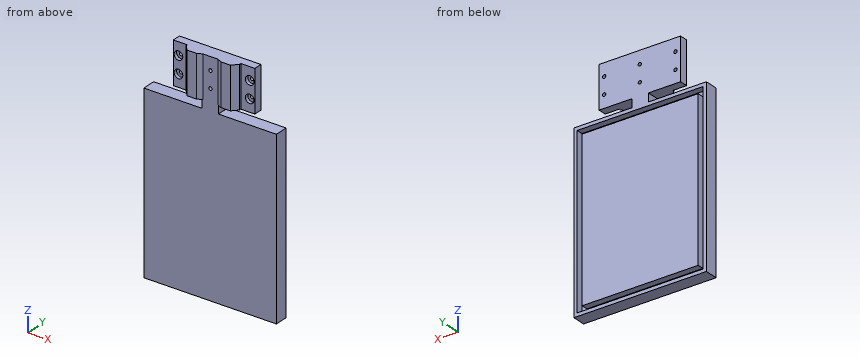
from build123d import *

# Parameters (mm, degrees)
BOSS_EXTRUDE2_DEPTH = 25.3
SKETCH3_R           = 1
CUT_EXTRUDE1_DEPTH  = 37.183559803
SKETCH4_R           = 1
CUT_EXTRUDE2_DEPTH  = 36.640566774
SKETCH5_R           = 2.6
CUT_EXTRUDE3_DEPTH  = 2
SKETCH7_W           = 10
SKETCH7_H           = 8
BOSS_EXTRUDE4_DEPTH = 5
SKETCH8_W           = 80
SKETCH8_H           = 8
BOSS_EXTRUDE5_DEPTH = 105
SKETCH9_W           = 76
SKETCH9_H           = 101
SKETCH9_W_2         = 70
SKETCH9_H_2         = 95
CUT_EXTRUDE4_DEPTH  = 4


with BuildPart() as part:
    # Sketch2 → Boss-Extrude2 (new body)
    with BuildSketch(Plane.XY):
        Polygon((4.5, 3.4), (-4.5, 3.4), (-7.5, 2), (-13.1, 2), (-16.1, 5.4), (-16.1, 6.4), (-24.6, 6.4), (-24.6, 11.4), (24.6, 11.4), (24.6, 6.4), (16.1, 6.4), (16.1, 5.4), (13.1, 2), (7.5, 2), align=None)
    extrude(amount=BOSS_EXTRUDE2_DEPTH)

    # Sketch3 → Cut-Extrude1 (cut, through all)
    with BuildSketch(Plane.XZ.offset(-3.4)):
        with Locations(Location((0, 17.55, 0), (0, 0, 270))):
            Circle(SKETCH3_R)
        with Locations(Location((0, 7.55, 0), (0, 0, 90))):
            Circle(SKETCH3_R)
    extrude(amount=-CUT_EXTRUDE1_DEPTH, mode=Mode.SUBTRACT)

    # Sketch4 → Cut-Extrude2 (cut, through all)
    with BuildSketch(Plane.XZ.offset(-6.4)):
        with Locations(Location((-21.5, 17.65, 0), (0, 0, 270))):
            Circle(SKETCH4_R)
        with Locations(Location((21.5, 17.65, 0), (0, 0, 90))):
            Circle(SKETCH4_R)
        with Locations(Location((-21.5, 7.65, 0), (0, 0, 270))):
            Circle(SKETCH4_R)
        with Locations(Location((21.5, 7.65, 0), (0, 0, 90))):
            Circle(SKETCH4_R)
    extrude(amount=-CUT_EXTRUDE2_DEPTH, mode=Mode.SUBTRACT)

    # Sketch5 → Cut-Extrude3 (cut)
    with BuildSketch(Plane.XZ.offset(-6.4)):
        with Locations(Location((-21.5, 17.65, 0), (0, 0, 270))):
            Circle(SKETCH5_R)
        with Locations(Location((-21.5, 7.45, 0), (0, 0, 90))):
            Circle(SKETCH5_R)
        with Locations(Location((21.5, 7.45, 0), (0, 0, 270))):
            Circle(SKETCH5_R)
        with Locations(Location((21.5, 17.65, 0), (0, 0, 90))):
            Circle(SKETCH5_R)
    extrude(amount=-CUT_EXTRUDE3_DEPTH, mode=Mode.SUBTRACT)

    # Sketch7 → Boss-Extrude4 (add)
    with BuildSketch(Plane(origin=(0, 0, 0), x_dir=(-1, 0, 0), z_dir=(0, 0, -1))):
        with Locations((0.191701822, 7.4)):
            Rectangle(SKETCH7_W, SKETCH7_H)
    extrude(amount=BOSS_EXTRUDE4_DEPTH)

    # Sketch8 → Boss-Extrude5 (add)
    with BuildSketch(Plane(origin=(0, 0, -5), x_dir=(-1, 0, 0), z_dir=(0, 0, -1))):
        with Locations((0.191701822, 7.4)):
            Rectangle(SKETCH8_W, SKETCH8_H)
    extrude(amount=BOSS_EXTRUDE5_DEPTH)

    # Sketch9 → Cut-Extrude4 (cut)
    with BuildSketch(Plane(origin=(0, 11.4, 0), x_dir=(1, 0, 0), z_dir=(0, 1, 0))):
        with Locations((-0.191701822, 57.5)):
            Rectangle(SKETCH9_W, SKETCH9_H)
        with Locations((-0.191701822, 57.5)):
            Rectangle(SKETCH9_W_2, SKETCH9_H_2, mode=Mode.SUBTRACT)
    extrude(amount=-CUT_EXTRUDE4_DEPTH, mode=Mode.SUBTRACT)


solid = part.part
Design review of the part built by this model. Coordinates are the model's own, in mm. Coordinates: 2 decimals unless noted, no trailing zeros. Order: outer loops, then holes, each group sorted by start corner. A loop starts at its lowest first (then second) coordinate and runs counter-clockwise, first axis right, second up. Notation, with made-up numbers: (13.25, 9.25) -> (48.25, 9.25) arc R13 cw to (48.25, 16.25) -> close; hole circle Ø5 at (18.25, 31). An arc over 180 degrees is marked (long way). One line per item, written item: value.
1) We need section C-C, the plane x = 32. Give the boundary of the cut face in (y, z).
Output values:
outline: (3.4, -110) -> (11.4, -110) -> (11.4, -108) -> (7.4, -108) -> (7.4, -105) -> (11.4, -105) -> (11.4, -10) -> (7.4, -10) -> (7.4, -7) -> (11.4, -7) -> (11.4, -5) -> (3.4, -5) -> close
2) Clearance check with flat-ended pins moving along their axes: P1, Ø1.6, axis at x = -22, z = 18, coming from the -Y side; P2, Ø1.5, axis at y = 6.5, z = -2.5, coming from the +X side; P3, Ø6, axis at x = -21.5, z = 7.45, coming from the -Y side; P4, Ø2, axis at x = -21, y = 5.5, coming from the +Z side. State where each tip first meets the part, or that it passes through.
Output values:
P1: stops at y = 8.4
P2: stops at x = 4.81
P3: stops at y = 6.4
P4: stops at z = 25.3
3) We need section B-B, the plane z = -76.5. Give the boundary of the cut face in (x, y).
Output values:
outline: (-40.19, 3.4) -> (39.81, 3.4) -> (39.81, 11.4) -> (37.81, 11.4) -> (37.81, 7.4) -> (34.81, 7.4) -> (34.81, 11.4) -> (-35.19, 11.4) -> (-35.19, 7.4) -> (-38.19, 7.4) -> (-38.19, 11.4) -> (-40.19, 11.4) -> close
4) To check wall thickness, follow probe 1 along Z at (x, y) = (-8, 8.5); probe 2 along X at (y, z) = (7.75, 7.45); probe 3 along X at (y, z) = (10.75, -95). State the ranges of each line that lie inside material, in increasing order. Write a range as [from, to].
Output values:
probe 1: z = [-110, -108], [-105, -10], [-7, -5], [0, 25.3]
probe 2: x = [-24.6, -24.1], [-18.9, -0.99], [0.99, 18.9], [24.1, 24.6]
probe 3: x = [-40.19, -38.19], [-35.19, 34.81], [37.81, 39.81]
5) We need section A-A, the plane y = 10. Count the separate pieces of the cut face and the enclosed holes in it, then the cut area to 3 significant figures.
Output values:
separate pieces: 2
enclosed holes: 7
area: 8,650 mm2
